Check sheet for the modelled part. Datum: model origin and axes. Units: mm. A direction names the side the tool comes from. Coordinates: 2 decimals unless noted, no trailing zeros. Write each loop counter-clockwise with the first axis right and the second up, starting at its lowest first coordinate (ties: lowest second). Pieces come first, ordered by that corner, then holes. Notation, with made-up numbers: M -29,51.5 L 1,51.5 A12 ccw 1,67.5 Z; hole C -12,-13 d2. An arc over 180 degrees is marked long. Answer as CSV lines item,"result". Start each with the question number.
1) Material ranges on L1, parallel to X at y = 2.75, z = 0; L2, parallel to Z at x = -6, y = 12; L3, parallel to Y at x = -3.8, z = 0, recorded low to high. Write a range as [from, to].
2) Section check D-D (y = 7.5). Record the cut outline in (x, z), and give its area (3 significant figures).
3) Draft check along Z on faces 1 (the flat face through (7, 10, 0)), 2 (the cylindrical face through (-4.97, 15.14, -2.1)), 3 (the cylindrical face through (10, 2, 12)). Enter one of: +Z half, -Z half, draft (parallel to the pull), parting line (faces both ways), or undercut.
4) Section check A-A (z = 12). Record the cut outline in (x, y), and give its area (3 significant figures).
5) Access from +Z, -Z, +X, -X, +Y, -Y to the whole of each face (thin tool, end or side, straight path). Record for faces 4 (the flat face through (-1.1, 3.5, 3)), 5 (the flat face through (0, 4, 0)), 6 (the flat face through (-8, 4, -1)), 7 (the flat face through (2, 10, 0)), 8 (the cylindrical face through (-2.49, 14.44, -0.54)).
6) Go/stop test with flat-tipped pins: pin 1 Ø5 at (y, z) = (8.5, 0.5) entering from -X; pin 2 Ø4 at (y, z) = (10.5, 1) entering from +X; pin 3 Ø1.5 at (x, z) = (4.5, 10) entering from -Y; pin 4 Ø1.8 at (x, z) = (8, 8.5) entering from +Y. Record where each tip stops, or that it passes through.
7) Section check C-C (y = 12). Record the cut outline in (x, z), and give its area (3 significant figures).
from build123d import *
from build123d.topology import SkipClean

# Parameters (mm, degrees)
SKETCH2_W               = 14
SKETCH2_H               = 6
BOSS_EXTRUDE1_DEPTH     = 4
SKETCH3_W               = 4
SKETCH3_H               = 6
BOSS_EXTRUDE2_DEPTH     = 12
CUT_EXTRUDE1_DEPTH      = 22.470910554
CUT_EXTRUDE1_DEPTH_BACK = 22.470910554
SKETCH4_R               = 1.5
BOSS_EXTRUDE3_START     = 1
SKETCH5_R               = 2.5
SKETCH5_R_2             = 1.5
BOSS_EXTRUDE3_DEPTH     = 1
SKETCH6_R               = 2.5
SKETCH6_R_2             = 1.5
BOSS_EXTRUDE4_DEPTH     = 1
SKETCH7_R               = 1
SKETCH7_W               = 4
SKETCH7_H               = 6
BOSS_EXTRUDE5_DEPTH     = 4
FILLET1_R               = 2
FILLET2_R               = 3


with BuildPart() as part:
    # Sketch2 → Boss-Extrude1 (new body)
    with BuildSketch(Plane(origin=(0, 0, 0), x_dir=(1, 0, 0), z_dir=(0, 1, 0))):
        Rectangle(SKETCH2_W, SKETCH2_H)
    extrude(amount=BOSS_EXTRUDE1_DEPTH)

    # Sketch3 → Boss-Extrude2 (add)
    with BuildSketch(Plane(origin=(0, 4, 0), x_dir=(1, 0, 0), z_dir=(0, 1, 0))):
        with Locations((-5, 0)):
            Rectangle(SKETCH3_W, SKETCH3_H)
        with Locations((5, 0)):
            Rectangle(SKETCH3_W, SKETCH3_H)
    extrude(amount=BOSS_EXTRUDE2_DEPTH)

    # Sketch4 → Cut-Extrude1 (cut, two sides: drawn at the far end of the back side and taken through both)
    with BuildSketch(Plane(origin=(7, 0, 0), x_dir=(0, 0, -1), z_dir=(1, 0, 0)).offset(-CUT_EXTRUDE1_DEPTH_BACK)):
        with Locations((0, 12)):
            Circle(SKETCH4_R)
    extrude(amount=CUT_EXTRUDE1_DEPTH + CUT_EXTRUDE1_DEPTH_BACK, mode=Mode.SUBTRACT)

    # Sketch5 → Boss-Extrude3 (add)
    with BuildSketch(Plane(origin=(-3, 0, 0), x_dir=(0, 0, -1), z_dir=(1, 0, 0)).offset(BOSS_EXTRUDE3_START)):
        with Locations(Location((0, 12, 0), (0, 0, 180))):
            Circle(SKETCH5_R)
        with Locations((0, 12)):
            Circle(SKETCH5_R_2, mode=Mode.SUBTRACT)
    extrude(amount=-BOSS_EXTRUDE3_DEPTH)

    # Sketch6 → Boss-Extrude4 (add)
    with SkipClean():  # the faces are left unmerged after this step: merging them gives an invalid solid
        with BuildSketch(Plane.ZY.offset(-3)):
            with Locations((0, 12)):
                Circle(SKETCH6_R)
            with Locations((0, 12)):
                Circle(SKETCH6_R_2, mode=Mode.SUBTRACT)
        extrude(amount=BOSS_EXTRUDE4_DEPTH)

    # Sketch7 → Boss-Extrude5 (add)
    # profile 1 of 2: a face of its own
    with SkipClean():  # the faces are left unmerged after this step: merging them gives an invalid solid
        with BuildSketch(Plane(origin=(0, 4, 0), x_dir=(1, 0, 0), z_dir=(0, 1, 0))):
            Polygon((11, 3), (11, -3), (11, -11), (11, -15), (7, -15), (7, -11), (7, -3), (7, 3), align=None)
            with Locations(Location((9, -12, 0), (0, 0, 270))):
                Circle(SKETCH7_R, mode=Mode.SUBTRACT)
        # profile 2 of 2: a face of its own
        with BuildSketch(Plane(origin=(0, 4, 0), x_dir=(1, 0, 0), z_dir=(0, 1, 0))):
            with Locations((-9, 0)):
                Rectangle(SKETCH7_W, SKETCH7_H)
            with Locations(Location((-9, 0, 0), (0, 0, 270))):
                Circle(SKETCH7_R, mode=Mode.SUBTRACT)
        extrude(amount=-BOSS_EXTRUDE5_DEPTH)

    # Fillet1
    fillet1_edges = [part.edges().sort_by_distance(p)[0] for p in [
        (-11, 2, -3),
        (11, 2, -3),
        (-11, 2, 3),
        (7, 2, 3),
        (11, 2, 15),
        (7, 2, 15),
    ]]
    fillet(fillet1_edges, radius=FILLET1_R - 0.0001)  # a hair under: the kernel refuses the full size

    # Fillet2
    fillet2_edges = [part.edges().sort_by_distance(p)[0] for p in [
        (-5, 16, -3),
        (5, 16, -3),
        (5, 16, 3),
        (-5, 16, 3),
    ]]
    fillet(fillet2_edges, radius=FILLET2_R - 0.0001)  # a hair under: the kernel refuses the full size


solid = part.part
Results found:
1,L1,"x = [-11, -10], [-8, 11]"
1,L2,"z = [-3, -1.5], [1.5, 3]"
1,L3,"y = [0, 10.5], [13.5, 16]"
2,outline,"M -7,-3 L -3,-3 L -3,3 L -7,3 Z; M 3,-3 L 7,-3 L 7,3 L 3,3 Z"
2,area,"48.0 mm2"
3,face 1,"draft"
3,face 2,"-Z half"
3,face 3,"undercut"
4,outline,"M 7,0 L 8,0 L 8,4 L 7,4 Z; M 10,0 L 11,0 L 11,4 L 10,4 Z"
4,area,"8.00 mm2"
5,face 4,"+Z, -X, +Y"
5,face 5,"+Z, -Z"
5,face 6,"+Z, -Z, -X, +Y"
5,face 7,"+Z, -Z, +Y"
5,face 8,"none"
6,pin 1,"stops at x = -7"
6,pin 2,"stops at x = 7"
6,pin 3,"passes through"
6,pin 4,"stops at y = 4"
7,outline,"M -7,-3 L -3,-3 L -3,-2.5 L -2,-2.5 L -2,-1.5 L -7,-1.5 Z; M -7,1.5 L -2,1.5 L -2,2.5 L -3,2.5 L -3,3 L -7,3 Z; M 2,-2.5 L 3,-2.5 L 3,-3 L 7,-3 L 7,-1.5 L 2,-1.5 Z; M 2,1.5 L 7,1.5 L 7,3 L 3,3 L 3,2.5 L 2,2.5 Z"
7,area,"28.0 mm2"
